Here's the drawing with two shaded views (mm, measured from the low corner). I have some questions. Give positions to 0.01 mm unless a question says otherwise; leave off trailing zeros. Loops run counter-clockwise (first coordinate to the right, second up) from the corner with the lowest first, then second, coordinate; pieces in that order, holes last. Notation, with made-up numbers: M -20,-36.75 L -14,-36.75 A18 cw -14,-19.75 Z; hole C 44.5,41.25 d2. An arc over 180 degrees is marked long. Use a Markdown table: item, result. Add a question column.
1) Suppose I cut it at A-A on y = 50. List the corners of the cut face in (x, z) for me.
2) Suppose I cut it at B-B on x = 11.5. List the corners of the cut face in (y, z) for me.
3) Suppose I cut it at C-C on z = 2.1. List the corners of the cut face in (x, y) for me, and give its area (3 significant figures).
4) Will this pin go through, and if not, where does the flat tip stop? pin 1 Ø1.5 at (x, z) = (82, 1.5) entering from -Y.
5) If I drill on line 1 along X through (y, z) = (120, 1.05); line 2 along Y through (x, z) = (74, 2.3); line 3 along Y through (x, z) = (5.5, 1.65), over which ranges is the centre line in solid material (lowest first)? Write a range as [from, to].
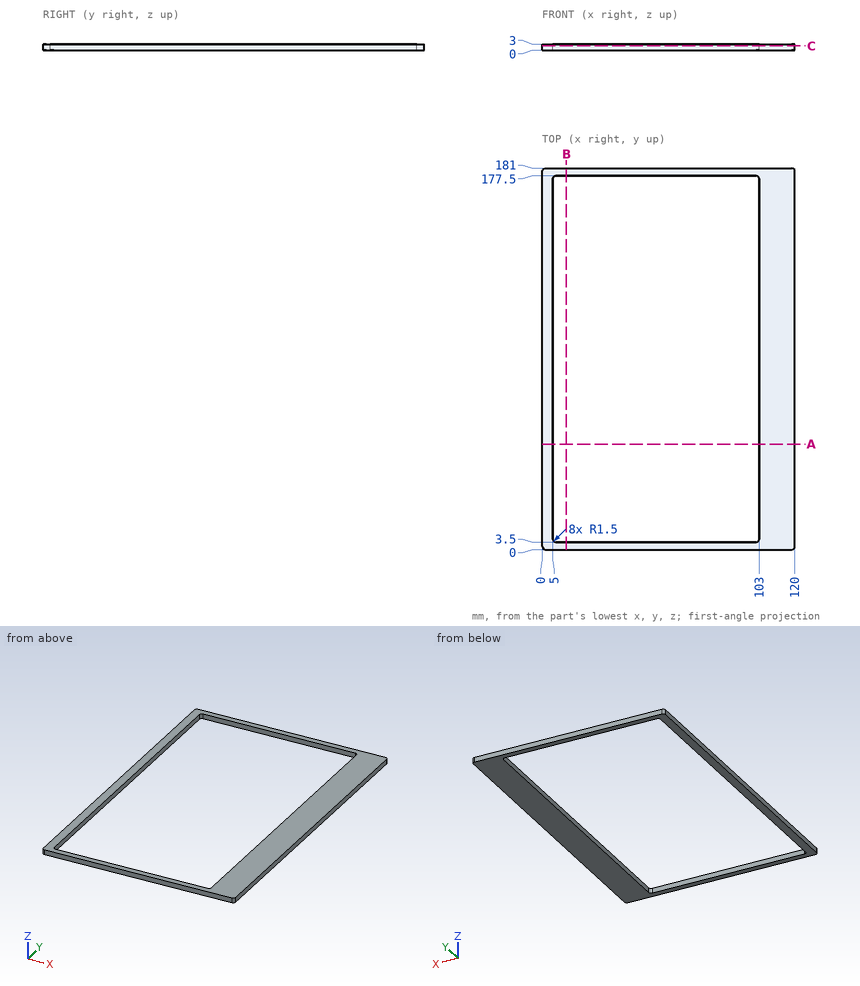
Answer block:
| question | item | result |
|---|---|---|
| 1 | outline | M 0,0 L 5,0 L 5,3 L 0,3 Z; M 103,0 L 120,0 L 120,3 L 103,3 Z |
| 2 | outline | M 0,0 L 3.5,0 L 3.5,3 L 0,3 Z; M 177.5,0 L 181,0 L 181,3 L 177.5,3 Z |
| 3 | outline | M 0,1.5 A1.5 ccw 1.5,0 L 118.5,0 A1.5 ccw 120,1.5 L 120,179.5 A1.5 ccw 118.5,181 L 1.5,181 A1.5 ccw 0,179.5 Z; hole M 5,5 A1.5 ccw 6.5,3.5 L 101.5,3.5 A1.5 ccw 103,5 L 103,176 A1.5 ccw 101.5,177.5 L 6.5,177.5 A1.5 ccw 5,176 Z |
| 3 | area | 4,670 mm^2 |
| 4 | pin 1 | stops at y = 0 |
| 5 | line 1 | x = [0, 5], [103, 120] |
| 5 | line 2 | y = [0, 3.5], [177.5, 181] |
| 5 | line 3 | y = [0, 3.88], [177.12, 181] |
